```python
from build123d import *

# Parameters (mm, degrees)
BOSS_EXTRUDE1_DEPTH = 5
SKETCH2_R           = 2.5
CUT_EXTRUDE1_DEPTH  = 125.526031415


with BuildPart() as part:
    # Model → Boss-Extrude1 (new body)
    with BuildSketch(Plane.XY):
        Polygon((-59.94, -89.08), (-59.93, -89.07), (-59.92, -89.05), (-59.91, -89.04), (-59.9, -89.02), (-59.9, -84.1), (-20.1, -84.1), (-20.1, -89.02), (-20.08, -89.06), (-20.07, -89.07), (-20.05, -89.08), (-20.04, -89.09), (-20.02, -89.1), (20.02, -89.1), (20.06, -89.08), (20.07, -89.07), (20.08, -89.05), (20.09, -89.04), (20.1, -89.02), (20.1, -84.1), (59.9, -84.1), (59.9, -89.02), (59.92, -89.06), (59.93, -89.07), (59.95, -89.08), (59.96, -89.09), (59.98, -89.1), (86.77, -89.1), (86.81, -89.08), (86.82, -89.07), (86.83, -89.05), (86.84, -89.04), (86.85, -89.02), (86.85, -59.98), (86.83, -59.94), (86.82, -59.93), (86.8, -59.92), (86.79, -59.91), (86.77, -59.9), (81.85, -59.9), (81.85, -20.1), (86.77, -20.1), (86.81, -20.08), (86.82, -20.07), (86.83, -20.05), (86.84, -20.04), (86.85, -20.02), (86.85, 20.02), (86.83, 20.06), (86.82, 20.07), (86.8, 20.08), (86.79, 20.09), (86.77, 20.1), (81.85, 20.1), (81.85, 59.9), (86.77, 59.9), (86.81, 59.92), (86.82, 59.93), (86.83, 59.95), (86.84, 59.96), (86.85, 59.98), (86.85, 89.02), (86.83, 89.06), (86.82, 89.07), (86.8, 89.08), (86.79, 89.09), (86.77, 89.1), (59.98, 89.1), (59.94, 89.08), (59.93, 89.07), (59.92, 89.05), (59.91, 89.04), (59.9, 89.02), (59.9, 84.1), (20.1, 84.1), (20.1, 89.02), (20.08, 89.06), (20.07, 89.07), (20.05, 89.08), (20.04, 89.09), (20.02, 89.1), (-20.02, 89.1), (-20.06, 89.08), (-20.07, 89.07), (-20.08, 89.05), (-20.09, 89.04), (-20.1, 89.02), (-20.1, 84.1), (-59.9, 84.1), (-59.9, 89.02), (-59.92, 89.06), (-59.93, 89.07), (-59.95, 89.08), (-59.96, 89.09), (-59.98, 89.1), (-86.77, 89.1), (-86.81, 89.08), (-86.82, 89.07), (-86.83, 89.05), (-86.84, 89.04), (-86.85, 89.02), (-86.85, 59.98), (-86.83, 59.94), (-86.82, 59.93), (-86.8, 59.92), (-86.79, 59.91), (-86.77, 59.9), (-81.85, 59.9), (-81.85, 20.1), (-86.77, 20.1), (-86.81, 20.08), (-86.82, 20.07), (-86.83, 20.05), (-86.84, 20.04), (-86.85, 20.02), (-86.85, -20.02), (-86.83, -20.06), (-86.82, -20.07), (-86.8, -20.08), (-86.79, -20.09), (-86.77, -20.1), (-81.85, -20.1), (-81.85, -59.9), (-86.77, -59.9), (-86.81, -59.92), (-86.82, -59.93), (-86.83, -59.95), (-86.84, -59.96), (-86.85, -59.98), (-86.85, -89.02), (-86.83, -89.06), (-86.82, -89.07), (-86.8, -89.08), (-86.79, -89.09), (-86.77, -89.1), (-59.98, -89.1), align=None)
    extrude(amount=BOSS_EXTRUDE1_DEPTH)

    # Sketch2 → Cut-Extrude1 (cut, through all)
    with BuildSketch(Plane.XY.offset(5)):
        with Locations((-45, 45)):
            Circle(SKETCH2_R)
        with Locations((-15, 45)):
            Circle(SKETCH2_R)
        with Locations((15, 45)):
            Circle(SKETCH2_R)
        with Locations((45, 45)):
            Circle(SKETCH2_R)
        with Locations((-15, 15)):
            Circle(SKETCH2_R)
        with Locations((15, 15)):
            Circle(SKETCH2_R)
        with Locations((45, 15)):
            Circle(SKETCH2_R)
        with Locations((-15, -15)):
            Circle(SKETCH2_R)
        with Locations((15, -15)):
            Circle(SKETCH2_R)
        with Locations((45, -15)):
            Circle(SKETCH2_R)
        with Locations((-15, -45)):
            Circle(SKETCH2_R)
        with Locations((15, -45)):
            Circle(SKETCH2_R)
        with Locations((45, -45)):
            Circle(SKETCH2_R)
        with Locations((-45, 15)):
            Circle(SKETCH2_R)
        with Locations((-45, -15)):
            Circle(SKETCH2_R)
        with Locations((-45, -45)):
            Circle(SKETCH2_R)
    extrude(amount=-CUT_EXTRUDE1_DEPTH, mode=Mode.SUBTRACT)


solid = part.part
```
For this review, take the finished solid that the model builds, in its own axes (mm). A direction names the side the tool comes from. Give positions to 0.01 mm unless a question says otherwise; leave off trailing zeros. Write each loop counter-clockwise with the first axis right and the second up, starting at its lowest first coordinate (ties: lowest second). Pieces come first, ordered by that corner, then holes. Notation, with made-up numbers: M 52,63 L 98,63 A17 ccw 98,91 Z; hole C 23.25,18 d6. An arc over 180 degrees is marked long. Answer as a JSON object with one key per item and string values. Group by question number.
Item 1: Draft analysis for pull direction X (two halves, no side actions). For faces 6 (the cylindrical face through (12.5, 15.1, 2.5)), 7 (the flat face through (74, 89.1, 2)), 8 (the flat face through (-86.85, 75, 2)), state which applies: +X half, -X half, draft (parallel to the pull), parting line (faces both ways), or undercut.
Item 2: Consider section D-D on x = -24. Write out the cut boundary in (y, z), plus the area to 3 significant figures.
Item 3: Consider section C-C on z = 3.7. Count the separate pieces of the cut face and the enclosed holes in it, plus the area to 3 significant figures.
Item 4: Consider section A-A on x = 15. Write out the cut boundary in (y, z).
Item 5: For probe 1 along Y at (x, z) = (-45, 3.5); probe 2 along Y at (x, z) = (-15, 2.1); probe 3 along Y at (x, z) = (-26, 4.75), list the stretches that pass through material, from the lowest coordinate up. Write a range as [from, to].
Item 6: Tool access review of faces 1 (the flat face through (-74, -89.1, 2)), 2 (the flat face through (59.9, 87, 2)), 3 (the flat face through (40, -84.1, 2)), 4 (the flat face through (84, -59.9, 2)), 5 (the flat face through (0, 89.1, 2)): name each direction out of +Z, -Z, +X, -X, +Y, -Y from which nothing blocks a thin tool from reaching the whole face with its end or side.
Item 7: Consider section B-B on y = 45. Write out the cut boundary in (x, z), plus the area to 4 significant figures.
Item 8: For pin 1 Ø6 at (x, y) = (-45, 45) entering from +Z; pin 2 Ø1.5 at (x, z) = (33.5, 1.5) entering from -Y; pin 3 Ø4 at (x, y) = (15, 45) entering from -Z, all flat-tipped, find the tip position at first contact; note any pin that passes through.
Check result:
{
 "1": {"face 6": "undercut", "face 7": "draft", "face 8": "-X half"},
 "2": {"outline": "M -84.1,0 L 84.1,0 L 84.1,5 L -84.1,5 Z", "area": "841 mm^2"},
 "3": {"separate pieces": "1", "enclosed holes": "16", "area": "29,000 mm^2"},
 "4": {"outline": "M -89.1,0 L -47.5,0 L -47.5,5 L -89.1,5 Z; M -42.5,0 L -17.5,0 L -17.5,5 L -42.5,5 Z; M -12.5,0 L 12.5,0 L 12.5,5 L -12.5,5 Z; M 17.5,0 L 42.5,0 L 42.5,5 L 17.5,5 Z; M 47.5,0 L 89.1,0 L 89.1,5 L 47.5,5 Z"},
 "5": {"probe 1": "y = [-84.1, -47.5], [-42.5, -17.5], [-12.5, 12.5], [17.5, 42.5], [47.5, 84.1]", "probe 2": "y = [-89.1, -47.5], [-42.5, -17.5], [-12.5, 12.5], [17.5, 42.5], [47.5, 89.1]", "probe 3": "y = [-84.1, 84.1]"},
 "6": {"face 1": "+Z, -Z, +X, -X, -Y", "face 2": "+Z, -Z, +Y", "face 3": "+Z, -Z, -Y", "face 4": "+Z, -Z, +X", "face 5": "+Z, -Z, +X, -X, +Y"},
 "7": {"outline": "M -81.85,0 L -47.5,0 L -47.5,5 L -81.85,5 Z; M -42.5,0 L -17.5,0 L -17.5,5 L -42.5,5 Z; M -12.5,0 L 12.5,0 L 12.5,5 L -12.5,5 Z; M 17.5,0 L 42.5,0 L 42.5,5 L 17.5,5 Z; M 47.5,0 L 81.85,0 L 81.85,5 L 47.5,5 Z", "area": "718.5 mm^2"},
 "8": {"pin 1": "stops at z = 5", "pin 2": "stops at y = -84.1", "pin 3": "passes through"}
}
